Input: part model. Units: mm. Frame: model coordinates. Face numbers are marked on the shaded views. A direction names the side the tool comes from. Give positions to 0.01 mm unless a question says otherwise; leave off trailing zeros. Write each loop counter-clockwise with the first axis right and the second up, starting at its lowest first coordinate (ties: lowest second). Pieces come first, ordered by that corner, then holes.
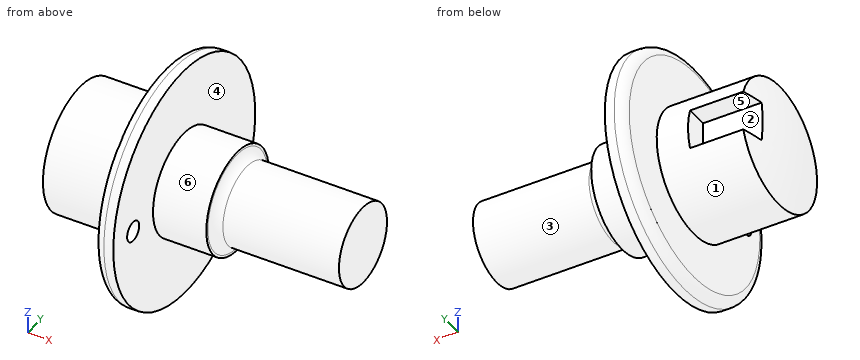
```python
from build123d import *

# Parameters (mm, degrees)
FILETE1_R             = 3
ESBO_O2_W             = 12.7
ESBO_O2_H             = 16
CORTE_EXTRUS_O1_DEPTH = 20
ESBO_O3_R             = 3.175
CORTE_EXTRUS_O2_DEPTH = 20


with BuildPart() as part:
    # Esboço1 → Revolução1 (revolve)
    with BuildSketch(Plane.XY, mode=Mode.PRIVATE) as revolu_o1_sk:
        with BuildLine():
            Line((45.5, 12.7), (8.5, 12.7))
            ThreePointArc((8.5, 12.7), (6.378679656, 13.578679656), (5.5, 15.7))
            Line((5.5, 15.7), (5.5, 16.5))
            Line((5.5, 16.5), (-11.5, 16.5))
            Line((-11.5, 16.5), (-11.5, 37.5))
            Line((-11.5, 37.5), (-17.5, 37.5))
            Line((-17.5, 37.5), (-17.5, 20))
            Line((-17.5, 20), (-44.5, 20))
            ThreePointArc((-44.5, 20), (-46.745828054, 10.111874208), (-47.5, 0))
            Line((-47.5, 0), (47.5, 0))
            ThreePointArc((47.5, 0), (46.996937848, 6.428257929), (45.5, 12.7))
        make_face()
    revolve(revolu_o1_sk.sketch.rotate(Axis((-47.5, 0, 0), (1, 0, 0)), 90), axis=Axis((-47.5, 0, 0), (1, 0, 0)))  # turned: the seam where the file's is

    # Filete1
    filete1_edges = [part.edges().sort_by_distance(p)[0] for p in [
        (-17.5, 0, -37.5),
    ]]
    fillet(filete1_edges, radius=FILETE1_R)

    # Esboço2 → Corte-extrusão1 (cut)
    with BuildSketch(Plane.ZY.offset(47.5)):
        with Locations((0, 20)):
            Rectangle(ESBO_O2_W, ESBO_O2_H)
    extrude(amount=-CORTE_EXTRUS_O1_DEPTH, mode=Mode.SUBTRACT)

    # Esboço3 → Corte-extrusão2 (cut)
    with BuildSketch(Plane.ZY.offset(17.5)):
        with Locations((0, -27)):
            Circle(ESBO_O3_R)
    extrude(amount=-CORTE_EXTRUS_O2_DEPTH, mode=Mode.SUBTRACT)


solid = part.part
```
Q1. Section D-D, the plane x = -25. Return the cut outline in (y, z), then the cut area to 3 significant figures.
Q2. Section B-B, the plane y = 0. Return the cut outline in (x, z) (1 decimal).
Q3. Pin query (flat end, axial travel): pin 1 (5.5 mm diameter, centred on y = -27, z = 0, fed in from -X); pin 2 (3 mm diameter, centred on y = -29.5, z = 22.5, fed in from +X); pin 3 (2 mm diameter, centred on x = 34, y = -8, fed in from -Z); pin 4 (6 mm diameter, centred on y = -12.5, z = -21.5, fed in from -X). Return the tip coordinate at first contact, or that it passes through.
Q4. Section A-A, the plane z = 0. Return the cut outline in (x, y) (1 decimal), then the cut area to 3 significant figures.
Q5. Section C-C, the plane x = 36.5. Return the cut outline in (y, z), then the cut area to 3 significant figures.
Q6. Material intervals for line 1 along Y through (x, z) = (-13.9, 0) (3 decimals); line 2 along Z through (x, y) = (27.5, 0.5); line 3 along Y through (x, z) = (-15.95, 0) (3 decimals), sorted ascending.
Q7. Access query for the marked faces 1, 2 and 3. Directions: +Z, -Z, +X, -X, +Y, -Y. A direction counts if a zero-diameter tool reaches every point of the face in a straight line with its end or side. Return the directions, or none.
Q8. Mould query, pull axis Z, two halves, no side actions, for the marked faces 4, 5 and 6. Classes: +Z half, -Z half, draft (parallel to the pull), parting line (faces both ways), or undercut.
Solutions:
1. outline: circle Ø40 at (0, 0)
1. area: 1,260 mm2
2. outline: (-44.5, -20) - (-17.5, -20) - (-17.5, -34.5) arc R3 ccw to (-14.5, -37.5) - (-11.5, -37.5) - (-11.5, -16.5) - (5.5, -16.5) - (5.5, -15.7) arc R3 cw to (8.5, -12.7) - (45.5, -12.7) arc R41.3 ccw to (45.5, 12.7) - (8.5, 12.7) arc R3 cw to (5.5, 15.7) - (5.5, 16.5) - (-11.5, 16.5) - (-11.5, 37.5) - (-14.5, 37.5) arc R3 ccw to (-17.5, 34.5) - (-17.5, 20) - (-44.5, 20) arc R68.2 ccw to start
3. pin 1: passes through
3. pin 2: stops at x = -11.5
3. pin 3: stops at z = -10.6
3. pin 4: stops at x = -17.5
4. outline: (-46.4, 12) arc R68.2 ccw to (-44.5, -20) - (-17.5, -20) - (-17.5, -23.8) - (-11.5, -23.8) - (-11.5, -16.5) - (5.5, -16.5) - (5.5, -15.7) arc R3 cw to (8.5, -12.7) - (45.5, -12.7) arc R41.3 ccw to (45.5, 12.7) - (8.5, 12.7) arc R3 cw to (5.5, 15.7) - (5.5, 16.5) - (-11.5, 16.5) - (-11.5, 37.5) - (-14.5, 37.5) arc R3 ccw to (-17.5, 34.5) - (-17.5, 20) - (-27.5, 20) - (-27.5, 12) - close; (-17.5, -34.5) arc R3 ccw to (-14.5, -37.5) - (-11.5, -37.5) - (-11.5, -30.2) - (-17.5, -30.2) - close
4. area: 3,040 mm2
5. outline: circle Ø25.4 at (0, 0)
5. area: 507 mm2
6. line 1: y = -37.5 to -30.175, -23.825 to 37.5
6. line 2: z = -12.69 to 12.69
6. line 3: y = -37.126 to -30.175, -23.825 to 37.126
7. face 1: -X
7. face 2: -X, +Y
7. face 3: +X
8. face 4: draft
8. face 5: undercut
8. face 6: parting line
